Here's how the part is built. I have some questions about the finished solid (model axes, mm). Give positions to 0.01 mm unless a question says otherwise; leave off trailing zeros. Order: outer loops, then holes, each group sorted by start corner. A loop starts at its lowest first (then second) coordinate and runs counter-clockwise, first axis right, second up. Notation, with made-up numbers: M 1.5,48 L 51.5,48 A14 cw 51.5,58 Z; hole C 72,28.25 d3. An arc over 180 degrees is marked long. Use one line per item in the form item = value.
from build123d import *

# Parameters (mm, degrees)
F2_R     = 10
F2_R_2   = 8
F3_DEPTH = 20
F4_R     = 1
F5_R     = 1


with BuildPart() as f3:
    # F2 (on Top) → F3 (new body)
    with BuildSketch(Plane.XY):
        Circle(F2_R)
        Circle(F2_R_2, mode=Mode.SUBTRACT)
    extrude(amount=F3_DEPTH)

    # F4
    f4_edges = [f3.edges().sort_by_distance(p)[0] for p in [
        (-8, 0, 20),
    ]]
    fillet(f4_edges, radius=F4_R)

    # F5
    f5_edges = [f3.edges().sort_by_distance(p)[0] for p in [
        (-8, 0, 0),
    ]]
    fillet(f5_edges, radius=F5_R)


solid = f3.part
Q1. I want a section at A-A on x = 0. Write out the boundary of the cut face in (y, z).
Found:
outline = M -10,0 L -9,0 A1 ccw -8,1 L -8,19 A1 ccw -9,20 L -10,20 Z; M 8,1 A1 ccw 9,0 L 10,0 L 10,20 L 9,20 A1 ccw 8,19 Z
Q2. I'm going to push flat-ended pins straight in: pin 1 Ø2 at (y, z) = (-7, 6.5) entering from -X; pin 2 Ø5 at (x, y) = (-4.5, -4.5) entering from +Z; pin 3 Ø5 at (y, z) = (1.5, 8.5) entering from +X; pin 4 Ø9.5 at (x, y) = (0, 0) entering from +Z. Where does each tip first touch, or does it pass through?
Found:
pin_1 = -8
pin_2 = 19.99
pin_3 = 10
pin_4 = through
Q3. Thinking about a two-plate mould opening in Y: for faces 1 (the face through (-9, 2, 0)), 2 (the face through (-1.73, -7.81, 9.87)), 3 (the face through (-2.17, -9.76, 9.86)), which applies, +Y half, -Y half, draft (parallel to the pull), parting line (faces both ways), or undercut?
Found:
face_1 = draft
face_2 = undercut
face_3 = parting line
Q4. I need wall thicknesses on L1, parallel to Y at x = 0, z = 6.5; L2, parallel to Y at x = 1, z = 16.5; L3, parallel to X at y = -5.5, z = 4.25. Which ranges of each line are inside material? Lowest first, please.
Found:
L1 = -10 to -8, 8 to 10
L2 = -9.95 to -7.94, 7.94 to 9.95
L3 = -8.35 to -5.81, 5.81 to 8.35
Q5. I want a section at C-C on z = 8.5. Write out the boundary of the cut face in (x, y), then the cut area to 3 significant figures.
Found:
outline = C 0,0 d20; hole C 0,0 d16
area = 113 mm²
